from build123d import *

# Parameters (mm, degrees)
BOSS_EXTRUDE1_DEPTH           = 15
TAP_DRILL_FOR_M2_5_TAP1_D     = 2.05
TAP_DRILL_FOR_M2_5_TAP1_DEPTH = 11.5


with BuildPart() as part:
    # Sketch1 → Boss-Extrude1 (new body)
    with BuildSketch(Plane.XY):
        Polygon((-1.299038106, 2.25), (-2.598076211, 0), (-1.299038106, -2.25), (1.299038106, -2.25), (2.598076211, 0), (1.299038106, 2.25), align=None)
    extrude(amount=BOSS_EXTRUDE1_DEPTH)

    # Tap Drill for M2.5 Tap1
    with Locations(Plane.XY.offset(15)):
        with Locations((0, 0)):
            Hole(TAP_DRILL_FOR_M2_5_TAP1_D / 2, depth=TAP_DRILL_FOR_M2_5_TAP1_DEPTH)


solid = part.part
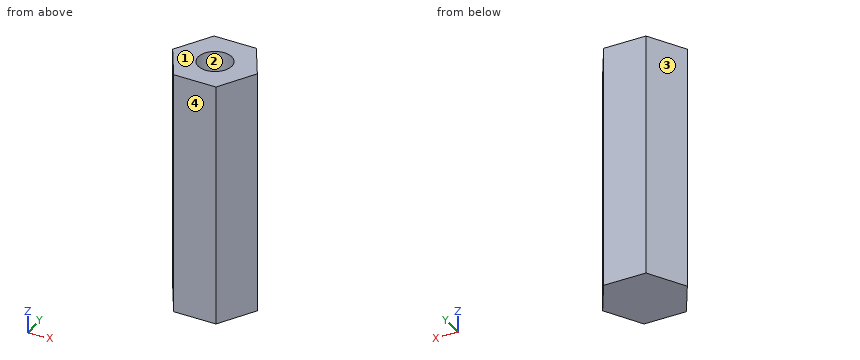
The listing builds one solid part. Answer for the finished solid, in the listing's coordinates (mm). Face numbers are marked on the shaded views. Give positions to 0.01 mm unless a question says otherwise; leave off trailing zeros. Loops run counter-clockwise (first coordinate to the right, second up) from the corner with the lowest first, then second, coordinate; pieces in that order, holes last. Notation, with made-up numbers: M -31.75,-33.75 L -7.75,-33.75 A21 cw -7.75,-21.75 Z; hole C 0.5,43 d3. An arc over 180 degrees is marked long. Answer as CSV lines item,"result".
Item 1: Straight lines are drawn through the part: line 1 along Y through (x, z) = (0, 10) (3 decimals); line 2 along Z through (x, y) = (-0.7, 0.25); line 3 along Y through (x, z) = (-0.65, 11.5). For each, find the intervals that lie inside material, in ascending order. Write a range as [from, to].
Values follow:
line 1,"y = [-2.25, -1.025], [1.025, 2.25]"
line 2,"z = [0, 3.5]"
line 3,"y = [-2.25, -0.79], [0.79, 2.25]"
Item 2: The mould has two halves that part along Y. Classify the marked faces 1, 2, 3 and 4: released by +Y, released by -Y, zero draft, split by the parting line, or undercut.
Values follow:
face 1,"zero draft"
face 2,"undercut"
face 3,"released by +Y"
face 4,"released by -Y"
Item 3: The part is cut by section A-A (z = 10). Give the vertices of the cut face in (x, y) (3 decimals).
Values follow:
outline,"M -2.598,0 L -1.299,-2.25 L 1.299,-2.25 L 2.598,0 L 1.299,2.25 L -1.299,2.25 Z; hole C 0,0 d2.05"
Item 4: The part is cut by section D-D (x = 1.9). Give the vertices of the cut face in (y, z), and give its area (3 significant figures).
Values follow:
outline,"M -1.21,0 L 1.21,0 L 1.21,15 L -1.21,15 Z"
area,"36.3 mm^2"
Item 5: The part is cut by section B-B (x = 0). Give the vertices of the cut face in (y, z) (3 decimals), and give its area (3 significant figures).
Values follow:
outline,"M -2.25,0 L 2.25,0 L 2.25,15 L 1.025,15 L 1.025,3.5 L -1.025,3.5 L -1.025,15 L -2.25,15 Z"
area,"43.9 mm^2"
Item 6: Given pin 1 Ø1.5 at (y, z) = (-0.5, 2.5) entering from -X; pin 2 Ø1.6 at (x, y) = (0, 0) entering from +Z; pin 3 Ø1 at (y, z) = (-1, 5) entering from -X, each flat-ended and moving along its own axis, determine where each tip first touches the part or whether it passes through.
Values follow:
pin 1,"stops at x = -2.6"
pin 2,"stops at z = 3.5"
pin 3,"stops at x = -2.31"
Item 7: The part is cut by section C-C (y = 1.6). Give the vertices of the cut face in (x, z), and give its area (3 significant figures).
Values follow:
outline,"M -1.67,0 L 1.67,0 L 1.67,15 L -1.67,15 Z"
area,"50.2 mm^2"
